Could you check a few things on this model? Use its own coordinates, in mm. A direction names the side the tool comes from. Give positions to 0.01 mm unless a question says otherwise; leave off trailing zeros. Order: outer loops, then holes, each group sorted by start corner. A loop starts at its lowest first (then second) coordinate and runs counter-clockwise, first axis right, second up. Notation, with made-up numbers: M -35.75,89 L -25.75,89 A25 ccw -25.75,123 Z; hole C 43.5,-2 d11. An arc over 180 degrees is marked long. Use a Markdown table: item, result. Add a question column.
```python
from build123d import *

# Parameters (mm, degrees)
SKETCH1_W           = 77.8
SKETCH1_H           = 59.9
BOSS_EXTRUDE1_DEPTH = 21.5
CUT_EXTRUDE1_DEPTH  = 75.588672062
FILLET1_R           = 2
SKETCH4_W           = 73.8
SKETCH4_H           = 17.3
CUT_EXTRUDE2_DEPTH  = 20
SKETCH5_R           = 1.75
CUT_EXTRUDE3_DEPTH  = 54.011437445
SKETCH6_W           = 0.3
SKETCH6_H           = 1
BOSS_EXTRUDE2_DEPTH = 3.2


with BuildPart() as part:
    # Sketch1 → Boss-Extrude1 (new body)
    with BuildSketch(Plane.XY):
        Rectangle(SKETCH1_W, SKETCH1_H)
    extrude(amount=BOSS_EXTRUDE1_DEPTH)

    # Sketch2 → Cut-Extrude1 (cut, through all)
    with BuildSketch(Plane.XZ.offset(29.95)):
        Polygon((-36.9, 21.5), (36.9, 21.5), (36.9, 18), (29, 18), (23, 12), (12, 12), (12, 6), (-12, 6), (-12, 12), (-23, 12), (-29, 18), (-36.9, 18), align=None)
    extrude(amount=-CUT_EXTRUDE1_DEPTH, mode=Mode.SUBTRACT)

    # Fillet1
    fillet1_edges = [part.edges().sort_by_distance(p)[0] for p in [
        (-12, 0, 12),
        (-23, 0, 12),
        (-29, 0, 18),
        (-36.9, 0, 18),
        (36.9, 0, 18),
        (29, 0, 18),
        (23, 0, 12),
        (12, 0, 12),
        (12, 0, 6),
        (-12, 0, 6),
    ]]
    fillet(fillet1_edges, radius=FILLET1_R)

    # Sketch4 → Cut-Extrude2 (cut)
    with BuildSketch(Plane.XY.offset(21.5)):
        with Locations((0, 19.3)):
            Rectangle(SKETCH4_W, SKETCH4_H)
        Rectangle(SKETCH4_W, SKETCH4_H)
        with Locations((0, -19.3)):
            Rectangle(SKETCH4_W, SKETCH4_H)
    extrude(amount=-CUT_EXTRUDE2_DEPTH, mode=Mode.SUBTRACT)

    # Sketch5 → Cut-Extrude3 (cut, through all)
    with BuildSketch(Plane.XY.offset(1.5)):
        with Locations((-27.9, 0)):
            Circle(SKETCH5_R)
        with Locations((-27.9, 19.3)):
            Circle(SKETCH5_R)
        with Locations(Location((27.9, 0, 0), (0, 0, 180))):
            Circle(SKETCH5_R)
        with Locations(Location((27.9, 19.3, 0), (0, 0, 180))):
            Circle(SKETCH5_R)
        with Locations((27.9, -19.3)):
            Circle(SKETCH5_R)
        with Locations(Location((-27.9, -19.3, 0), (0, 0, 180))):
            Circle(SKETCH5_R)
    extrude(amount=-CUT_EXTRUDE3_DEPTH, mode=Mode.SUBTRACT)

    # Sketch6 → Boss-Extrude2 (add)
    with BuildSketch(Plane(origin=(0, 0, 0), x_dir=(-1, 0, 0), z_dir=(0, 0, -1))):
        with Locations((-36, 0)):
            Rectangle(SKETCH6_W, SKETCH6_H)
        with Locations((-36, 19.3)):
            Rectangle(SKETCH6_W, SKETCH6_H)
        with Locations((36, 19.3)):
            Rectangle(SKETCH6_W, SKETCH6_H)
        with Locations((36, 0)):
            Rectangle(SKETCH6_W, SKETCH6_H)
        with Locations((36, -19.3)):
            Rectangle(SKETCH6_W, SKETCH6_H)
        with Locations((-36, -19.3)):
            Rectangle(SKETCH6_W, SKETCH6_H)
    extrude(amount=BOSS_EXTRUDE2_DEPTH)


solid = part.part
```
1) Suppose I cut it at A-A on x = 34. Please give me the cut outline in (y, z), and give its area (3 significant figures).
2) Suppose I cut it at B-B on y = -7. Please give me the cut outline in (x, z), and give its area (3 significant figures).
3) For pin 1 (8 mm diameter, centred on x = 0.5, y = 2.5, fed in from -Z); pin 2 (0.8 mm diameter, centred on y = -19.5, z = -1.5, fed in from -X); pin 3 (2 mm diameter, centred on x = 27.9, y = -19.3, fed in from -Z); pin 4 (1 mm diameter, centred on x = 33, y = 9.5, fed in from +Z), each with a flat end and sliding along its axis, tell me the tip position at first contact or that it passes through.
4) Suppose I cut it at C-C on x = -13. Please give me the cut outline in (y, z), and give its area (3 significant figures).
5) Please list where these lines run through material, in increasing order: line 1 (Y direction, x = -27, z = 6.75); line 2 (X direction, y = 14, z = 17.5). Write a range as from..to.
6) We'd pull the mould along X, two halves only. Please class faces 1 (the face through (26, 10, 15)), 2 (the face through (-0.5, 29.95, 5.8)): pulls with the +X half, pulls with the -X half, needs draft (parallel to the pull), parting line crosses it, or undercut.
7) For faces 3 (the face through (-18, -10, 12)), 4 (the face through (-1, 0, 1.5)), 5 (the face through (-0.5, -29.95, 5.8)), which set-ups out of +Z, -Z, +X, -X, +Y, -Y let a thin tool reach every point of the face, with its end or its side?
Values found:
| question | item | result |
|---|---|---|
| 1 | outline | M -29.95,0 L 29.95,0 L 29.95,18 L 27.95,18 L 27.95,1.5 L 10.65,1.5 L 10.65,18 L 8.65,18 L 8.65,1.5 L -8.65,1.5 L -8.65,18 L -10.65,18 L -10.65,1.5 L -27.95,1.5 L -27.95,18 L -29.95,18 Z |
| 1 | area | 222 mm^2 |
| 2 | outline | M -38.9,0 L 38.9,0 L 38.9,21.5 L 36.9,21.5 L 36.9,1.5 L -36.9,1.5 L -36.9,21.5 L -38.9,21.5 Z |
| 2 | area | 197 mm^2 |
| 3 | pin 1 | stops at z = 0 |
| 3 | pin 2 | stops at x = -36.15 |
| 3 | pin 3 | passes through |
| 3 | pin 4 | stops at z = 18 |
| 4 | outline | M -29.95,0 L 29.95,0 L 29.95,11.73 L 27.95,11.73 L 27.95,1.5 L 10.65,1.5 L 10.65,11.73 L 8.65,11.73 L 8.65,1.5 L -8.65,1.5 L -8.65,11.73 L -10.65,11.73 L -10.65,1.5 L -27.95,1.5 L -27.95,11.73 L -29.95,11.73 Z |
| 4 | area | 172 mm^2 |
| 5 | line 1 | y = -29.95..-27.95, -10.65..-8.65, 8.65..10.65, 27.95..29.95 |
| 5 | line 2 | x = -38.9..-36.9, 36.9..38.9 |
| 6 | face 1 | undercut |
| 6 | face 2 | needs draft |
| 7 | face 3 | +Z, +Y, -Y |
| 7 | face 4 | +Z |
| 7 | face 5 | +Z, -Z, +X, -X, -Y |
